Here's how the part is built. I have some questions about the finished solid (model axes, mm). A direction names the side the tool comes from. Round coordinates to 2 decimals unless told otherwise and drop trailing zeros. Loops run counter-clockwise (first coordinate to the right, second up) from the corner with the lowest first, then second, coordinate; pieces in that order, holes last. Notation, with made-up numbers: (28.25, 78.25) - (56.25, 78.25) arc R25 ccw to (56.25, 100.25) - close; hole circle Ø6 at (81, -3). An arc over 180 degrees is marked (long way). Answer as a JSON object with one key per item and string values. Group by question number.
1) If we mould it in two halves opening along X, with no side actions, what happens to faces 5 (the face through (199.012, -166.868, 75.57)), 6 (the face through (128, -25, 304.8)), 7 (the face through (234.07, -25.04, 272.42)), 8 (the face through (33.97, -25.044, 19.503))? For each: pulls with the +X half, pulls with the -X half, needs draft (parallel to the pull), parting line crosses it, or undercut.
2) I want a section at D-D, the plane x = 143. Please give me the cut outline in (y, z), then the cut area to 3 significant figures.
3) If I drill on line 1 along X through (y, z) = (-39, 266); line 2 along Z through (x, y) = (215.9, -30); line 3 along Z through (x, y) = (38.1, -13), over which ranges is the centre line in solid material (lowest first)? Write a range as [from, to].
4) I want a section at A-A, the plane y = -78.5. Please give me the cut outline in (x, z).
5) I want a section at B-B, the plane y = -24. Please give me the cut outline in (x, z), then the cut area to 3 significant figures.
6) I want a section at C-C, the plane z = 281.5. Please give me the cut outline in (x, y).
7) Will these pins go through, and if not, where does the flat tip stop? P1, Ø10, axis at x = 112.5, z = 130, coming from the -Y side; P2, Ø12, axis at y = -134, z = 70, coming from the -X side; P3, Ø1, axis at x = 111.5, z = 73.5, coming from the -Y side.
8) Which directions (+Z, -Z, +X, -X, +Y, -Y) give clear straight access to the entire face, cutting with the end or side of a thin tool? Please do faces 1 (the face through (124, -62.484, 149)), 2 (the face through (220.82, -96.75, 66.39)), 3 (the face through (37.36, -95.13, 236.75)), 4 (the face through (11.46, -25.04, 293.94)).
from build123d import *

# Parameters (mm, degrees)
F0_R     = 19.05
F1_DEPTH = 50.8
F2_DEPTH = 62.484
F3_DEPTH = 125.222
F5_DEPTH = 44.45
F7_DEPTH = 44.45
F8_DEPTH = 299.212


with BuildPart() as f1:
    # F0 (on Front) → F1 (new body)
    with BuildSketch(Plane.XZ):
        with BuildLine():
            ThreePointArc((0, 38.1), (11.1592316368, 11.1592316368), (38.1, 0))
            Line((38.1, 0), (215.9, 0))
            ThreePointArc((215.9, 0), (242.8407683632, 11.1592316368), (254, 38.1))
            Line((254, 38.1), (254, 266.7))
            ThreePointArc((254, 266.7), (242.8407683632, 293.6407683632), (215.9, 304.8))
            Line((215.9, 304.8), (38.1, 304.8))
            ThreePointArc((38.1, 304.8), (11.1592316368, 293.6407683632), (0, 266.7))
            Line((0, 266.7), (0, 38.1))
        make_face()
        with Locations((38.1, 38.1)):
            Circle(F0_R, mode=Mode.SUBTRACT)
        Polygon((243.3144801542, 88.8824801542), (184.404, 29.972), (152.9731035763, 61.4028964237), (38.9238964237, 175.4521035763), (7.493, 206.883), (66.4034801542, 265.7934801542), (97.834376578, 234.3625837305), (211.8835837305, 120.313376578), align=None, mode=Mode.SUBTRACT)
        with Locations((215.9, 266.7)):
            Circle(F0_R, mode=Mode.SUBTRACT)
    extrude(amount=F1_DEPTH)

    # F0 (on Front) → F2 (join)
    with BuildSketch(Plane.XZ):
        Polygon((38.9238964237, 175.4521035763), (152.9731035763, 61.4028964237), (211.8835837305, 120.313376578), (97.834376578, 234.3625837305), align=None)
    extrude(amount=F2_DEPTH)

    # F0 (on Front) → F3 (join)
    with BuildSketch(Plane.XZ):
        Polygon((152.9731035763, 61.4028964237), (184.404, 29.972), (243.3144801542, 88.8824801542), (211.8835837305, 120.313376578), align=None)
        Polygon((7.493, 206.883), (38.9238964237, 175.4521035763), (97.834376578, 234.3625837305), (66.4034801542, 265.7934801542), align=None)
    extrude(amount=F3_DEPTH)

    # F4 (on face) → F5 (join)
    with BuildSketch(Plane(origin=(77.216, 0, -77.216), x_dir=(0, 1, 0), z_dir=(0.7071067812, 0, -0.7071067812))):
        with BuildLine():
            Line((-125.222, 151.5867233236), (-125.222, 234.8987233236))
            ThreePointArc((-125.222, 234.8987233236), (-166.878, 193.2427233236), (-125.222, 151.5867233236))
        make_face()
    extrude(amount=-F5_DEPTH)

    # F6 (on face) → F7 (join)
    with BuildSketch(Plane(origin=(-99.695, 0, 99.695), x_dir=(0, -1, 0), z_dir=(-0.7071067812, 0, 0.7071067812))):
        with BuildLine():
            Line((125.222, 164.0327233236), (125.222, 151.5867233236))
            ThreePointArc((125.222, 151.5867233236), (166.878, 193.2427233236), (125.222, 234.8987233236))
            Line((125.222, 234.8987233236), (125.222, 222.4527233236))
            ThreePointArc((125.222, 222.4527233236), (145.8765890785, 213.8973124021), (154.432, 193.2427233236))
            ThreePointArc((154.432, 193.2427233236), (145.8765890785, 172.5881342452), (125.222, 164.0327233236))
        make_face()
    extrude(amount=-F7_DEPTH)

    # F6 (on face) → F8 (cut)
    with BuildSketch(Plane(origin=(-99.695, 0, 99.695), x_dir=(0, -1, 0), z_dir=(-0.7071067812, 0, 0.7071067812))):
        with BuildLine():
            Line((125.222, 222.4527233236), (125.222, 164.0327233236))
            ThreePointArc((125.222, 164.0327233236), (145.8765890785, 172.5881342452), (154.432, 193.2427233236))
            ThreePointArc((154.432, 193.2427233236), (145.8765890785, 213.8973124021), (125.222, 222.4527233236))
        make_face()
        with BuildLine():
            ThreePointArc((125.222, 222.4527233236), (96.012, 193.2427233236), (125.222, 164.0327233236))
            Line((125.222, 164.0327233236), (125.222, 222.4527233236))
        make_face()
    extrude(amount=-F8_DEPTH, mode=Mode.SUBTRACT)


solid = f1.part
Outcome:
{
 "1": {"face 5": "parting line crosses it", "face 6": "needs draft", "face 7": "undercut", "face 8": "undercut"},
 "2": {"outline": "(-62.48, 71.38) - (-50.8, 71.38) - (-50.8, 0) - (0, 0) - (0, 304.8) - (-50.8, 304.8) - (-50.8, 189.2) - (-62.48, 189.2) - close", "area": "16,900 mm^2"},
 "3": {"line 1": "[0, 196.86], [234.94, 254]", "line 2": "[0, 247.65], [285.75, 304.8]", "line 3": "[0, 19.05], [57.15, 304.8]"},
 "4": {"outline": "(7.49, 206.88) - (38.92, 175.45) - (97.83, 234.36) - (66.4, 265.79) - close; (152.97, 61.4) - (184.4, 29.97) - (243.31, 88.88) - (211.88, 120.31) - close"},
 "5": {"outline": "(0, 38.1) arc R38.1 ccw to (38.1, 0) - (215.9, 0) arc R38.1 ccw to (254, 38.1) - (254, 266.7) arc R38.1 ccw to (215.9, 304.8) - (38.1, 304.8) arc R38.1 ccw to (0, 266.7) - close; hole circle Ø38.1 at (38.1, 38.1); hole circle Ø38.1 at (215.9, 266.7)", "area": "73,900 mm^2"},
 "6": {"outline": "(2.99, -50.8) - (203.91, -50.8) - (203.91, 0) - (2.99, 0) - close; (227.89, -50.8) - (251.01, -50.8) - (251.01, 0) - (227.89, 0) - close"},
 "7": {"P1": "y = -62.48", "P2": "x = 155.57", "P3": "y = -50.8"},
 "8": {"face 1": "-Y", "face 2": "-Z, +X, -Y", "face 3": "+Z, -X, -Y", "face 4": "+Z, -X, +Y, -Y"}
}
